Could you check a few things on this model? Use its own coordinates, in mm. Face numbers are marked on the shaded views. A direction names the side the tool comes from. Round coordinates to 2 decimals unless told otherwise and drop trailing zeros. Write each loop counter-clockwise with the first axis right and the second up, starting at its lowest first coordinate (ties: lowest second). Pieces come first, ordered by that corner, then holes. Notation, with made-up numbers: M 75,-19 L 94,-19 A23 ccw 94,11 Z; hole C 78,-16 d4. An arc over 180 degrees is marked long. One line per item, written item: value. Start each with the question number.
(1) I want a section at A-A on z = -31. Please give me the cut outline in (x, y), and give its area (3 significant figures).
(2) If I drill on L1, parallel to X at y = 28, z = -3.5; L2, parallel to Y at x = 40, z = -3; L3, parallel to X at y = 28, z = -0.15, over which ranges is the centre line in solid material (lowest first)?
(3) I want a section at D-D on x = 5. Please give me the cut outline in (y, z), and give its area (3 significant figures).
(4) Thinking about a two-plate mould opening in X: for the marked faces 1, 2, 3 and 4, which applies, released by +X, released by -X, zero draft, split by the parting line, or undercut?
(5) I want a section at C-C on z = -16.5. Please give me the cut outline in (x, y), and give its area (3 significant figures).
(6) Which directions (+Z, -Z, +X, -X, +Y, -Y) give clear straight access to the entire face, cutting with the end or side of a thin tool? Please do the marked faces 5, 6, 7 and 8.
(7) I want a section at B-B on x = 40. Please give me the cut outline in (y, z) (3 decimals), and give its area (4 significant figures).
(8) I'm going to push flat-ended pins straight in: pin 1 Ø4 at (x, z) = (54.5, -30.5) entering from +Y; pin 2 Ø3 at (y, z) = (13.5, -6) entering from -X; pin 3 Ø3 at (x, z) = (5, -31) entering from -Y; pin 4 Ø6.5 at (x, y) = (35, 23) entering from +Z. Where does each tip first touch, or does it pass through?
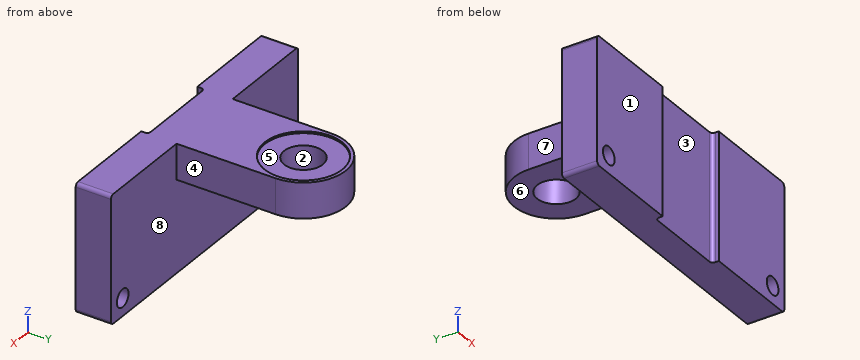
```python
from build123d import *

# Parameters (mm, degrees)
SKETCH_1_W          = 80
SKETCH_1_H          = 10
EXTRUDE_1_DEPTH     = 36
EXTRUDE_3_DEPTH     = 10
FILLET_1_RADIUS     = 12
FILLET_1_LENGTH     = 10
SKETCH_3_W          = 24
SKETCH_3_H          = 2
CUT_EXTRUDE_1_DEPTH = 97.415766346
SKETCH_6_R          = 2.5
CUT_EXTRUDE_2_DEPTH = 97.415766346
FILLET_2_R          = 1


with BuildPart() as part:
    # 草图1 → 凸台-拉伸1 (new body)
    with BuildSketch(Plane.XY):
        with Locations((40, -5)):
            Rectangle(SKETCH_1_W, SKETCH_1_H)
    extrude(amount=-EXTRUDE_1_DEPTH)

    # 草图2 → 凸台-拉伸3 (add)
    with BuildSketch(Plane.XY):
        Polygon((28, 0), (28, 40), (52, 40), (52, 0), (80, 0), (80, -10), (0, -10), (0, 0), align=None)
    extrude(amount=-EXTRUDE_3_DEPTH)

    # 圆角1: full round fillet: the end face becomes a half cylinder, R = half its width
    fillet_1_face = Plane((40, 40, -5), x_dir=(0, 0, 1), z_dir=(0, 1, 0))  # on the end face: x along it, z out of the body
    fillet_1_slab = fillet_1_face.offset(-FILLET_1_RADIUS / 2) * Box(FILLET_1_LENGTH, 2 * FILLET_1_RADIUS, FILLET_1_RADIUS, mode=Mode.PRIVATE)  # the body's end, R deep
    fillet_1_round = Plane((40, 28, -5), x_dir=(0, 1, 0), z_dir=(0, 0, 1)) * Cylinder(FILLET_1_RADIUS, FILLET_1_LENGTH, mode=Mode.PRIVATE)  # its axis R under the face
    add(fillet_1_slab - fillet_1_round, mode=Mode.SUBTRACT)

    # 草图3 → 切除-拉伸1 (cut, through all)
    with BuildSketch(Plane.XY):
        with Locations((40, -9)):
            Rectangle(SKETCH_3_W, SKETCH_3_H)
    extrude(amount=-CUT_EXTRUDE_1_DEPTH, mode=Mode.SUBTRACT)

    # 草图5 → M10 六角头螺栓C级的柱形沉头孔1 (revolve, cut)
    with BuildSketch(Plane(origin=(40, 28, 0), x_dir=(0, -1, 0), z_dir=(1, 0, 0))):
        Polygon((0, 0), (0, 36), (5.5, 36), (5.5, 0.5), (11, 0.5), (11, 0.020977491), (11.025, 0), align=None)
    revolve(axis=Axis((40, 28, 6.35), (0, 0, -1)), mode=Mode.SUBTRACT)

    # 草图6 → 切除-拉伸2 (cut, through all)
    with BuildSketch(Plane(origin=(0, 0, 0), x_dir=(1, 0, 0), z_dir=(0, 1, 0))):
        with Locations(Location((75, 31, 0), (0, 0, 270))):
            Circle(SKETCH_6_R)
        with Locations(Location((5, 31, 0), (0, 0, 270))):
            Circle(SKETCH_6_R)
    extrude(amount=-CUT_EXTRUDE_2_DEPTH, mode=Mode.SUBTRACT)

    # 圆角2
    fillet_2_edges = [part.edges().sort_by_distance(p)[0] for p in [
        (80, -5, -36),
        (0, -5, -36),
        (80, -5, 0),
        (28, -8, -18),
        (52, -8, -18),
        (0, -5, 0),
    ]]
    fillet(fillet_2_edges, radius=FILLET_2_R)


solid = part.part
```
Found:
1. outline: M 0,-10 L 2.5,-10 L 2.5,0 L 0,0 Z; M 7.5,-10 L 28,-10 L 28,-9 A1 cw 29,-8 L 51,-8 A1 cw 52,-9 L 52,-10 L 72.5,-10 L 72.5,0 L 7.5,0 Z; M 77.5,-10 L 80,-10 L 80,0 L 77.5,0 Z
1. area: 652 mm²
2. L1: x = 28 to 34.5, 45.5 to 52
2. L2: y = -8 to 22.5, 33.5 to 40
2. L3: x = 28 to 29, 51 to 52
3. outline: M -10,-36 L 0,-36 L 0,-33.5 L -10,-33.5 Z; M -10,-28.5 L 0,-28.5 L 0,0 L -10,0 Z
3. area: 310 mm²
4. face 1: zero draft
4. face 2: undercut
4. face 3: undercut
4. face 4: released by +X
5. outline: M 0,-10 L 28,-10 L 28,-9 A1 cw 29,-8 L 51,-8 A1 cw 52,-9 L 52,-10 L 80,-10 L 80,0 L 0,0 Z
5. area: 752 mm²
6. face 5: +Z
6. face 6: -Z, +X, -X, +Y
6. face 7: +Z, -Z, -X, +Y
6. face 8: -Z, +Y
7. outline: M -8,-36 L 0,-36 L 0,-10 L 22.5,-10 L 22.5,-0.5 L 17,-0.5 L 17,-0.021 L 16.975,0 L -8,0 Z; M 33.5,-10 L 40,-10 L 40,0 L 39.025,0 L 39,-0.021 L 39,-0.5 L 33.5,-0.5 Z
7. area: 572.5 mm²
8. pin 1: stops at y = 0
8. pin 2: stops at x = 28
8. pin 3: passes through
8. pin 4: stops at z = -0.5
